```python
from build123d import *

# Parameters (mm, degrees)
SKETCH1_R           = 6
BOSS_EXTRUDE1_DEPTH = 45.2
SHELL1_T            = -1.5
SKETCH2_R           = 3.5
BOSS_EXTRUDE2_DEPTH = 5.2
SHELL2_START        = -3.7
SHELL2_OUTLINE_R    = 2
SHELL2_DEPTH        = 5.2
SKETCH3_R           = 2.5
BOSS_EXTRUDE3_DEPTH = 6.1
SKETCH4_R           = 1.5
BOSS_EXTRUDE4_DEPTH = 6.1
SKETCH5_R           = 0.75
CUT_EXTRUDE1_DEPTH  = 12.1
SKETCH6_R           = 2
CUT_EXTRUDE2_DEPTH  = 12.1
SKETCH7_R           = 2.5
BOSS_EXTRUDE5_DEPTH = 8
SKETCH8_R           = 1.5
BOSS_EXTRUDE6_DEPTH = 6.1
SKETCH9_R           = 0.75
CUT_EXTRUDE3_DEPTH  = 14.1
SKETCH10_R          = 2
CUT_EXTRUDE4_DEPTH  = 14.1
BOSS_EXTRUDE7_START = -1.5
BOSS_EXTRUDE7_DEPTH = 1.5


# Read off the part's stored shape, not the designer's step: Shell2
with BuildPart() as part:
    # Sketch1 → Boss-Extrude1 (new body)
    with BuildSketch(Plane(origin=(0, 0, 0), x_dir=(1, 0, 0), z_dir=(0, 1, 0))):
        with Locations(Location((0, 0, 0), (0, 0, 270))):
            Circle(SKETCH1_R)
    extrude(amount=BOSS_EXTRUDE1_DEPTH)

    # Shell1
    shell1_openings = [part.faces().sort_by_distance(p)[0] for p in [
        (0, 45.2, 0),
    ]]
    offset(amount=SHELL1_T, openings=shell1_openings, kind=Kind.INTERSECTION)

    # Sketch2 → Boss-Extrude2 (add)
    with BuildSketch(Plane.XZ):
        with Locations(Location((0, 0, 0), (0, 0, 270))):
            Circle(SKETCH2_R)
    extrude(amount=BOSS_EXTRUDE2_DEPTH)

    # Shell2 outline → Shell2 (cut)
    with BuildSketch(Plane(origin=(0, 0, 0), x_dir=(1, 0, 0), z_dir=(0, 1, 0)).offset(SHELL2_START)):
        Circle(SHELL2_OUTLINE_R)
    extrude(amount=SHELL2_DEPTH, mode=Mode.SUBTRACT)

    # Sketch3 → Boss-Extrude3 (add)
    with BuildSketch(Plane.XY):
        with Locations(Location((0, -2.644163182, 0), (0, 0, 270))):
            Circle(SKETCH3_R)
    extrude(amount=BOSS_EXTRUDE3_DEPTH)

    # Sketch4 → Boss-Extrude4 (add)
    with BuildSketch(Plane.XY.offset(6.1)):
        with Locations((0, -2.644163182)):
            Circle(SKETCH4_R)
    extrude(amount=BOSS_EXTRUDE4_DEPTH)

    # Sketch5 → Cut-Extrude1 (cut)
    with BuildSketch(Plane.XY.offset(12.2)):
        with Locations((0, -2.644163182)):
            Circle(SKETCH5_R)
    extrude(amount=-CUT_EXTRUDE1_DEPTH, mode=Mode.SUBTRACT)

    # Sketch6 → Cut-Extrude2 (cut)
    with BuildSketch(Plane(origin=(0, -3.7, 0), x_dir=(1, 0, 0), z_dir=(0, 1, 0))):
        with Locations(Location((0, 0, 0), (0, 0, 270))):
            Circle(SKETCH6_R)
    extrude(amount=CUT_EXTRUDE2_DEPTH, mode=Mode.SUBTRACT)

    # Sketch7 → Boss-Extrude5 (add)
    with BuildSketch(Plane(origin=(0, 0, 0), x_dir=(0, 0, -1), z_dir=(1, 0, 0))):
        with Locations(Location((0, -2.644163182, 0), (0, 0, 188.130102354))):
            Circle(SKETCH7_R)
    extrude(amount=BOSS_EXTRUDE5_DEPTH)

    # Sketch8 → Boss-Extrude6 (add)
    with BuildSketch(Plane(origin=(8, 0, 0), x_dir=(0, 0, -1), z_dir=(1, 0, 0))):
        with Locations((0, -2.644163182)):
            Circle(SKETCH8_R)
    extrude(amount=BOSS_EXTRUDE6_DEPTH)

    # Sketch9 → Cut-Extrude3 (cut)
    with BuildSketch(Plane(origin=(14.1, 0, 0), x_dir=(0, 0, -1), z_dir=(1, 0, 0))):
        with Locations((0, -2.644163182)):
            Circle(SKETCH9_R)
    extrude(amount=-CUT_EXTRUDE3_DEPTH, mode=Mode.SUBTRACT)

    # Sketch10 → Cut-Extrude4 (cut)
    with BuildSketch(Plane(origin=(0, -3.7, 0), x_dir=(1, 0, 0), z_dir=(0, 1, 0))):
        with Locations(Location((0, 0, 0), (0, 0, 270))):
            Circle(SKETCH10_R)
    extrude(amount=CUT_EXTRUDE4_DEPTH, mode=Mode.SUBTRACT)

    # Sketch11 → Boss-Extrude7 (add)
    with BuildSketch(Plane(origin=(0, 45.2, 0), x_dir=(1, 0, 0), z_dir=(0, 1, 0)).offset(BOSS_EXTRUDE7_START)):
        with BuildLine():
            Line((3, -5.196152423), (3, -6.873863542))
            ThreePointArc((3, -6.873863542), (0, -7.5), (-3, -6.873863542))
            Line((-3, -6.873863542), (-3, -5.196152423))
            ThreePointArc((-3, -5.196152423), (0, -6), (3, -5.196152423))
        make_face()
        with BuildLine():
            Line((-3, 5.196152423), (-3, 6.873863542))
            ThreePointArc((-3, 6.873863542), (0, 7.5), (3, 6.873863542))
            Line((3, 6.873863542), (3, 5.196152423))
            ThreePointArc((3, 5.196152423), (0, 6), (-3, 5.196152423))
        make_face()
    extrude(amount=BOSS_EXTRUDE7_DEPTH)


solid = part.part
```
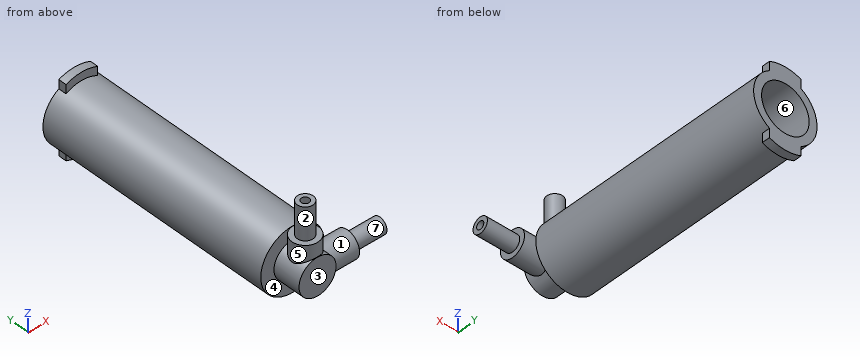
Work out the finished part from the listing and answer in its coordinate system (mm). Face numbers are marked on the shaded views. A direction names the side the tool comes from. Give positions to 0.01 mm unless a question says otherwise; leave off trailing zeros. Write each loop counter-clockwise with the first axis right and the second up, starting at its lowest first coordinate (ties: lowest second). Pieces come first, ordered by that corner, then holes.
(1) The mould has two halves that part along Y. Classify the marked faces 5, 6 and 7: pulls with the +Y half, pulls with the -Y half, needs draft (parallel to the pull), parting line crosses it, or undercut.
Final values:
face 5: undercut
face 6: needs draft
face 7: parting line crosses it
(2) The part is cut by section B-B on y = 8. Write down the section's boundary in (x, z), plus the area to 3 significant figures.
Final values:
outline: circle Ø12 at (0, 0); hole circle Ø9 at (0, 0)
area: 49.5 mm2
(3) The part is cut by section A-A on z = 3. Write down the section's boundary in (x, y).
Final values:
outline: (-5.2, 0) - (-1.8, 0) - (-1.8, -0.91) arc R2.5 ccw to (-1.8, -4.38) - (-1.8, -5.2) - (1.8, -5.2) - (1.8, -4.38) arc R2.5 ccw to (1.8, -0.91) - (1.8, 0) - (5.2, 0) - (5.2, 45.2) - (3.35, 45.2) - (3.35, 1.5) - (-3.35, 1.5) - (-3.35, 45.2) - (-5.2, 45.2) - close; hole circle Ø1.5 at (0, -2.64)
(4) Straight lines are drawn through the part: line 1 (X direction, y = -0.75, z = 0); line 2 (Z direction, x = 0, y = 14); line 3 (X direction, y = -1.6, z = 0). For each, find the intervals that lie inside material, in ascending order.
Final values:
line 1: x = -3.5 to -2, 2 to 8
line 2: z = -6 to -4.5, 4.5 to 6
line 3: x = -3.5 to -2, 2 to 14.1
(5) Which of the six approach directions +Z, -Z, +X, -X, +Y, -Y give full straight-line access (tool end or side, diameter ignored) to the marked faces 1, 2, 3 and 4?
Final values:
face 1: +X
face 2: +Z
face 3: +Z, -Z, +X, -X, -Y
face 4: none
(6) The part is cut by section C-C on x = 7. Write down the section's boundary in (y, z).
Final values:
outline: circle Ø5 at (-2.64, 0); hole circle Ø1.5 at (-2.64, 0)
(7) Flat-ended cylindrical pins translate along their axes: pin 1 Ø0.7 at (x, z) = (-0.5, -6) entering from -Y; pin 2 Ø10 at (x, y) = (-2.5, 2) entering from -Z; pin 3 Ø1.5 at (y, z) = (24.5, -2) entering from -X. Find the tip coordinate at first contact, or state that the pin passes through.
Final values:
pin 1: stops at y = 0
pin 2: stops at z = -6
pin 3: stops at x = -5.87
